CAD build for the part. Positions are in the model's coordinates, mm. A direction names the side the tool comes from. Give positions to 0.01 mm unless a question says otherwise; leave off trailing zeros. Write each loop counter-clockwise with the first axis right and the second up, starting at its lowest first coordinate (ties: lowest second). Pieces come first, ordered by that corner, then holes. Notation, with made-up numbers: (3.5, 35.25) -> (19.5, 35.25) arc R23 cw to (19.5, 69.25) -> close; hole circle Ø10 at (-39, -28). An arc over 180 degrees is marked (long way). Answer as a JSON object with one key per item and string values.
Autodesk Inventor part; units mm, degrees
ref_plane "YZ Plane" through (0, 0, 0) normal (1, 0, 0) x (0, 1, 0)
ref_plane "XZ Plane" through (0, 0, 0) normal (0, 1, 0) x (-1, 0, 0)
ref_plane "XY Plane" through (0, 0, 0) normal (0, 0, 1) x (1, 0, 0)
sketch "Sketch1" plane through (0, 0, 0) normal (0, 0, 1) x (1, 0, 0)
  line L0 (0, 19.2) -> (0, -14.4)
  line L1 (-14.4, 0) -> (19.2, 0)
  circle A0 centre (0, 0) radius 12
  dimension "d0" = 24
extrude "Extrusion1" add sketch "Sketch1" along normal mid plane 55
sketch "Sketch2" plane through (0, 0, 0) normal (0, 0, 1) x (1, 0, 0)
  circle A0 centre (0, 0) radius 12
  circle A1 centre (0, 0) radius 12
  circle A2 centre (0, 0) radius 10
  dimension "d3" = 20
extrude "Extrusion2" add sketch "Sketch2" along normal mid plane 78 contours A2
chamfer "Chamfer1" distance 2 angle 45 2 edges at (-10, 0, 39) (-10, 0, -39)
properties part number "Axle" material "Galvanized Steel"
1) Pin check, flat tips, straight feed: pin 1 (1 mm diameter, centred on y = -8.5, z = -16, fed in from -X); pin 2 (5 mm diameter, centred on x = -4.5, y = 8, fed in from -Z); pin 3 (12 mm diameter, centred on x = 7.5, z = -3.5, fed in from -Y); pin 4 (10 mm diameter, centred on x = 9.5, z = -18.5, fed in from -Y). Stop position of each tip, or through.
Model answer:
{"pin 1": "stops at x = -8.94", "pin 2": "stops at z = -39", "pin 3": "stops at y = -11.91", "pin 4": "stops at y = -11.12"}
2) Slice it at C-C (z = -34). List the corners of the cut face in (x, y).
Model answer:
{"outline": "circle Ø20 at (0, 0)"}
3) Slice it at D-D (z = 21). List the corners of the cut face in (x, y).
Model answer:
{"outline": "circle Ø24 at (0, 0)"}
4) Wall check: probe 1 along Z at (x, y) = (-5, -10); probe 2 along X at (y, z) = (-3.5, 3); probe 3 along X at (y, z) = (-3, -19). Give the ranges that are in metal, low to high.
Model answer:
{"probe 1": "z = -27.5 to 27.5", "probe 2": "x = -11.48 to 11.48", "probe 3": "x = -11.62 to 11.62"}
5) 3-axis set-ups, long thin cutter, end or side, ignore diameter. For faces 3 (the flat face through (0, 0, 39)), 4 (the cylindrical face through (-2.17, -9.76, -32.18)), 5 (the flat face through (-5, 9, 27.5)): which of +Z, -Z, +X, -X, +Y, -Y reach the whole face in a straight line?
Model answer:
{"face 3": "+Z, +X, -X, +Y, -Y", "face 4": "-Z", "face 5": "+Z"}
6) Slice it at A-A (y = 0). List the corners of the cut face in (x, z), then the cut area to 3 significant figures.
Model answer:
{"outline": "(-12, -27.5) -> (-10, -27.5) -> (-10, -37) -> (-8, -39) -> (8, -39) -> (10, -37) -> (10, -27.5) -> (12, -27.5) -> (12, 27.5) -> (10, 27.5) -> (10, 37) -> (8, 39) -> (-8, 39) -> (-10, 37) -> (-10, 27.5) -> (-12, 27.5) -> close", "area": "1,770 mm2"}
7) Mould opens along X. For faces 1 (the cylindrical face through (-2.17, 9.76, 32.18)), 2 (the flat face through (-5, 9, -27.5)) say: released by +X, released by -X, zero draft, split by the parting line, or undercut.
Model answer:
{"face 1": "split by the parting line", "face 2": "zero draft"}
